Here's how the part is built. I have some questions about the finished solid (model axes, mm). A direction names the side the tool comes from. Coordinates: 2 decimals unless noted, no trailing zeros. Write each loop counter-clockwise with the first axis right and the second up, starting at its lowest first coordinate (ties: lowest second). Pieces come first, ordered by that corner, then holes.
(1) Imagine slicing it at D-D, the plane y = -137. List the corners of the cut face in (x, z) for me, plus the area to 3 significant figures.
(2) Please list where these lines run through material, in increasing order: probe 1 along Y at (x, z) = (56, 6.5); probe 2 along X at (y, z) = (-117.5, 2); probe 3 along Y at (x, z) = (33, 5).
(3) For pin 1 Ø11 at (x, y) = (23.15, -88.54) entering from +Z; pin 2 Ø1 at (x, z) = (85, 7) entering from -Y; pin 3 Ø3 at (y, z) = (-127.5, 6.5) entering from -X, each with a flat end and sliding along its axis, tell me the tip position at first contact or that it passes through.
(4) Imagine slicing it at C-C, the plane z = 8. List the corners of the cut face in (x, y) for me.
(5) Imagine slicing it at B-B, the plane x = 81.5. List the corners of the cut face in (y, z) for me.
(6) Which directions (+Z, -Z, +X, -X, +Y, -Y) give clear straight access to the entire face, cutting with the end or side of a thin tool? Please do faces 4 (the flat face through (61.497, -106.333, 4.93)), 5 (the flat face through (40.55, -127.81, 4.93)).
(7) Thinking about a two-plate mould opening in X: for faces 1 (the flat face through (38.19, -57.94, 4.93)), 2 (the cylindrical face through (47.993, -113.811, 5.07)), 3 (the flat face through (42, -88, 10)), which applies, released by +X, released by -X, zero draft, split by the parting line, or undercut?
(8) Imagine slicing it at A-A, the plane y = -114. List the corners of the cut face in (x, z) for me.
```python
from build123d import *

# Parameters (mm, degrees)
BOSS_EXTRUDE1_DEPTH = 10
SKETCH2_R           = 7
CUT_EXTRUDE1_DEPTH  = 197.513344998


with BuildPart() as part:
    # Sketch1 → Boss-Extrude1 (new body)
    with BuildSketch(Plane.XY):
        with BuildLine():
            Line((5.549773739, -33.303117211), (5.549773739, -93.303117211))
            Line((5.549773739, -93.303117211), (76.549773739, -163.303117211))
            ThreePointArc((76.549773739, -163.303117211), (97.76244369, -163.152672743), (97.611999223, -141.940002792))
            Line((97.611999223, -141.940002792), (24.355880913, -69.715660797))
            Line((24.355880913, -69.715660797), (52.420485151, -45.825449879))
            ThreePointArc((52.420485151, -45.825449879), (52.86718031, -17.544706193), (24.586436624, -17.098011034))
            Line((24.586436624, -17.098011034), (5.549773739, -33.303117211))
        make_face()
    extrude(amount=BOSS_EXTRUDE1_DEPTH)

    # Sketch2 → Cut-Extrude1 (cut, through all)
    with BuildSketch(Plane.XY.offset(10)):
        with Locations((23.151883869, -88.542112922)):
            Circle(SKETCH2_R)
        with Locations((53.151883869, -118.542112922)):
            Circle(SKETCH2_R)
        with Locations((83.151883869, -148.542112922)):
            Circle(SKETCH2_R)
    extrude(amount=-CUT_EXTRUDE1_DEPTH, mode=Mode.SUBTRACT)


solid = part.part
```
Recorded:
1. outline: (49.87, 0) - (92.6, 0) - (92.6, 10) - (49.87, 10) - close
1. area: 427 mm2
2. probe 1: y = -143.04 to -124.94, -112.15 to -100.91, -41.15 to -21.77
2. probe 2: x = 30.09 to 46.23, 60.07 to 72.82
2. probe 3: y = -120.37 to -78.24, -62.36 to -12.23
3. pin 1: passes through
3. pin 2: stops at y = -167.54
3. pin 3: stops at x = 38.71
4. outline: (5.55, -93.3) - (76.55, -163.3) arc R15 ccw to (97.61, -141.94) - (24.36, -69.72) - (52.42, -45.83) arc R20 ccw to (24.59, -17.1) - (5.55, -33.3) - close; hole circle Ø14 at (23.15, -88.54); hole circle Ø14 at (53.15, -118.54); hole circle Ø14 at (83.15, -148.54)
5. outline: (-166.54, 0) - (-155.34, 0) - (-155.34, 10) - (-166.54, 10) - close; (-141.74, 0) - (-126.05, 0) - (-126.05, 10) - (-141.74, 10) - close
6. face 4: +Z, -Z, +X
6. face 5: +Z, -Z, -X, -Y
7. face 1: released by +X
7. face 2: undercut
7. face 3: zero draft
8. outline: (26.54, 0) - (47.83, 0) - (47.83, 10) - (26.54, 10) - close; (58.48, 0) - (69.27, 0) - (69.27, 10) - (58.48, 10) - close
